from build123d import *

# Parameters (mm, degrees)
F0_R      = 14.5
F1_DEPTH  = 10
F2_R      = 11.5
F3_DEPTH  = 9
F4_SIZE   = 0.5
F5_R      = 5.25
F6_DEPTH  = 12.5
F7_SIZE   = 0.5
F8_R      = 3.75
F9_DEPTH  = 8
F10_SIZE  = 0.5
F11_R     = 14.5
F11_R_2   = 11.5
F12_DEPTH = 6
F13_R     = 25
F14_DEPTH = 9
F15_SIZE  = 0.5
F16_R     = 2.75
F17_DEPTH = 19


with BuildPart() as f1:
    # F0 (on Top) → F1 (new body)
    with BuildSketch(Plane.XY):
        Circle(F0_R)
    extrude(amount=F1_DEPTH)

    # F2 (on face) → F3 (join)
    with BuildSketch(Plane.XY.offset(10)):
        Circle(F2_R)
        with BuildLine():
            ThreePointArc((-7.4852813742, 6.6310302931), (-5, 8.6602540378), (-2, 9.7979589711))
            Line((-2, 9.7979589711), (-2, 8.3))
            Line((-2, 8.3), (2, 8.3))
            Line((2, 8.3), (2, 9.7979589711))
            ThreePointArc((2, 9.7979589711), (5, 8.6602540378), (7.4852813742, 6.6310302931))
            Line((7.4852813742, 6.6310302931), (6.1880108514, 5.8820508076))
            Line((6.1880108514, 5.8820508076), (8.1880108514, 2.4179491924))
            Line((8.1880108514, 2.4179491924), (9.4852813742, 3.166928678))
            ThreePointArc((9.4852813742, 3.166928678), (10, 0), (9.4852813742, -3.166928678))
            Line((9.4852813742, -3.166928678), (8.1880108514, -2.4179491924))
            Line((8.1880108514, -2.4179491924), (6.1880108514, -5.8820508076))
            Line((6.1880108514, -5.8820508076), (7.4852813742, -6.6310302931))
            ThreePointArc((7.4852813742, -6.6310302931), (5, -8.6602540378), (2, -9.7979589711))
            Line((2, -9.7979589711), (2, -8.3))
            Line((2, -8.3), (-2, -8.3))
            Line((-2, -8.3), (-2, -9.7979589711))
            ThreePointArc((-2, -9.7979589711), (-5, -8.6602540378), (-7.4852813742, -6.6310302931))
            Line((-7.4852813742, -6.6310302931), (-6.1880108514, -5.8820508076))
            Line((-6.1880108514, -5.8820508076), (-8.1880108514, -2.4179491924))
            Line((-8.1880108514, -2.4179491924), (-9.4852813742, -3.166928678))
            ThreePointArc((-9.4852813742, -3.166928678), (-10, 0), (-9.4852813742, 3.166928678))
            Line((-9.4852813742, 3.166928678), (-8.1880108514, 2.4179491924))
            Line((-8.1880108514, 2.4179491924), (-6.1880108514, 5.8820508076))
            Line((-6.1880108514, 5.8820508076), (-7.4852813742, 6.6310302931))
        make_face(mode=Mode.SUBTRACT)
    extrude(amount=F3_DEPTH)

    # F4
    f4_edges = [f1.edges().sort_by_distance(p)[0] for p in [
        (0, 8.3, 19),
        (-7.188011, 4.15, 19),
        (-7.188011, -4.15, 19),
        (0, -8.3, 19),
        (7.188011, -4.15, 19),
        (7.188011, 4.15, 19),
    ]]
    chamfer(f4_edges, length=F4_SIZE)

    # F5 (on face) → F6 (join)
    with BuildSketch(Plane.XY.offset(10)):
        Circle(F5_R)
    extrude(amount=F6_DEPTH)

    # F7
    f7_edges = [f1.edges().sort_by_distance(p)[0] for p in [
        (-5.25, 0, 22.5),
    ]]
    chamfer(f7_edges, length=F7_SIZE)

    # F8 (on face) → F9 (join)
    with BuildSketch(Plane.XY.offset(22.5)):
        Circle(F8_R)
    extrude(amount=F9_DEPTH)

    # F10
    f10_edges = [f1.edges().sort_by_distance(p)[0] for p in [
        (-3.75, 0, 30.5),
    ]]
    chamfer(f10_edges, length=F10_SIZE)

    # F11 (on face) → F12 (join)
    with BuildSketch(Plane.XY.offset(10)):
        Circle(F11_R)
        Circle(F11_R_2, mode=Mode.SUBTRACT)
    extrude(amount=F12_DEPTH)

    # F13 (on face) → F14 (cut)
    with BuildSketch(Plane(origin=(0, 0, 0), x_dir=(1, 0, 0), z_dir=(0, 0, -1))):
        Circle(F13_R)
    extrude(amount=-F14_DEPTH, mode=Mode.SUBTRACT)

    # F15
    f15_edges = [f1.edges().sort_by_distance(p)[0] for p in [
        (-11.5, 0, 19),
        (-14.5, 0, 16),
        (-14.5, 0, 9),
    ]]
    chamfer(f15_edges, length=F15_SIZE)

    # F16 (on face) → F17 (cut)
    with BuildSketch(Plane.XY.offset(30.5)):
        Circle(F16_R)
    extrude(amount=-F17_DEPTH, mode=Mode.SUBTRACT)


solid = f1.part
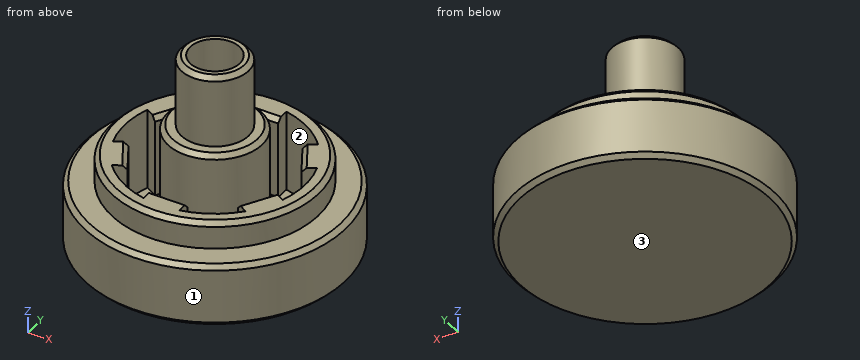
Build history of the part. All positions in model axes, mm. Face numbers are marked on the shaded views. Round coordinates to 2 decimals unless told otherwise and drop trailing zeros. Write each loop counter-clockwise with the first axis right and the second up, starting at its lowest first coordinate (ties: lowest second). Pieces come first, ordered by that corner, then holes. Notation, with made-up numbers: M 29.5,7 L 74.5,7 A10 ccw 74.5,12 Z; hole C 63,34 d4. An arc over 180 degrees is marked long. Answer as a JSON object with one key per item and string values. Group by question number.
(1) Cut at C-C (z = 23.5). Give the cut face in (x, y), and give its area (3 significant figures).
(2) Drill centre lines: L1, parallel to Y at x = 0, z = 17.25; L2, parallel to Z at x = -5, y = -4; L3, parallel to Z at x = 1.25, y = 11.5. Where is each one in solid material? Low to high.
(3) Mould opens along X. For the marked faces 1, 2 and 3 say: pulls with the +X half, pulls with the -X half, needs draft (parallel to the pull), parting line crosses it, or undercut.
(4) Cut at D-D (z = 21). Give the cut face in (x, y), and give its area (3 significant figures).
(5) Cut at A-A (z = 17.5). Give the cut face in (x, y), and give its area (3 significant figures).
(6) Flat gauge pins, fed straight in: pin 1 (10 mm diameter, centred on x = 3, y = -10.5, fed in from +Z); pin 2 (6 mm diameter, centred on x = -1, z = 25, fed in from +Y); pin 3 (1.2 mm diameter, centred on y = 9.5, z = 16.5, fed in from -X). Where does each tip first touch, or does it go through?
Responses:
{
 "1": {"outline": "C 0,0 d7.5; hole C 0,0 d5.5", "area": "20.4 mm2"},
 "2": {"L1": "y = -11.5 to -8.3, -5.25 to -2.75, 2.75 to 5.25, 8.3 to 11.5", "L2": "z = 9 to 10", "L3": "z = 9 to 16"},
 "3": {"face 1": "parting line crosses it", "face 2": "undercut", "face 3": "needs draft"},
 "4": {"outline": "C 0,0 d10.5; hole C 0,0 d5.5", "area": "62.8 mm2"},
 "5": {"outline": "C 0,0 d23; C 0,0 d10.5; hole M -9.49,-3.17 L -8.19,-2.42 L -6.19,-5.88 L -7.49,-6.63 A10 ccw -2,-9.8 L -2,-8.3 L 2,-8.3 L 2,-9.8 A10 ccw 7.49,-6.63 L 6.19,-5.88 L 8.19,-2.42 L 9.49,-3.17 A10 ccw 9.49,3.17 L 8.19,2.42 L 6.19,5.88 L 7.49,6.63 A10 ccw 2,9.8 L 2,8.3 L -2,8.3 L -2,9.8 A10 ccw -7.49,6.63 L -6.19,5.88 L -8.19,2.42 L -9.49,3.17 A10 ccw Z; hole C 0,0 d5.5", "area": "203 mm2"},
 "6": {"pin 1": "stops at z = 19", "pin 2": "stops at y = 5.19", "pin 3": "stops at x = -10.58"}
}
